```python
from build123d import *

# Parameters (mm, degrees)
F0_R     = 2.35
F0_R_2   = 0.6
F0_W     = 11.2562068871
F0_H     = 4.6791491237
F1_DEPTH = 25


with BuildPart() as f1:
    # F0 (on Top) → F1 (new body)
    with BuildSketch(Plane.XY):
        with BuildLine():
            Line((14.3979561755, 29.7439676553), (-32.8092921048, 29.7439676553))
            ThreePointArc((-32.8092921048, 29.7439676553), (-38.1665301992, 27.2495197857), (-39.7056679646, 21.5439676553))
            Line((-39.7056679646, 21.5439676553), (21.2943320354, 21.5439676553))
            ThreePointArc((21.2943320354, 21.5439676553), (19.7551942699, 27.2495197857), (14.3979561755, 29.7439676553))
        make_face()
        with Locations((-26.7056679646, 25.0439676553)):
            Circle(F0_R, mode=Mode.SUBTRACT)
        with Locations((-22.2056679646, 25.0439676553)):
            Circle(F0_R_2, mode=Mode.SUBTRACT)
        with BuildLine():
            ThreePointArc((-14.2060092107, 24.2939676534), (-14.0292525699, 24.2207333822), (-13.9560402329, 24.0439676553))
            ThreePointArc((-13.9560402329, 24.0439676553), (-14.3828278959, 23.8672019284), (-14.2060092107, 24.2939676534))
        make_face(mode=Mode.SUBTRACT)
        with BuildLine():
            ThreePointArc((-13.4558540993, 25.5439676553), (-13.6755569185, 25.0136046664), (-14.2059471661, 24.7939676611))
            ThreePointArc((-14.2059471661, 24.7939676611), (-14.9558540936, 25.5440607221), (-14.2057610325, 26.2939676495))
            ThreePointArc((-14.2057610325, 26.2939676495), (-13.6754911104, 26.0742648361), (-13.4558540993, 25.5439676553))
        make_face(mode=Mode.SUBTRACT)
        with BuildLine():
            ThreePointArc((-13.9556679658, 27.0439676553), (-14.0289022388, 26.8671799923), (-14.205698988, 26.7939676572))
            ThreePointArc((-14.205698988, 26.7939676572), (-14.3824336927, 27.2207553183), (-13.9556679658, 27.0439676553))
        make_face(mode=Mode.SUBTRACT)
        with BuildLine():
            ThreePointArc((-13.2056679646, 24.0439676553), (-12.9556679646, 24.2939676553), (-12.7056679646, 24.0439676553))
            ThreePointArc((-12.7056679646, 24.0439676553), (-12.9556679646, 23.7939676553), (-13.2056679646, 24.0439676553))
        make_face(mode=Mode.SUBTRACT)
        with BuildLine():
            ThreePointArc((-11.9557127462, 24.0439676553), (-11.7057127462, 24.2939676553), (-11.4557127462, 24.0439676553))
            ThreePointArc((-11.4557127462, 24.0439676553), (-11.7057127462, 23.7939676553), (-11.9557127462, 24.0439676553))
        make_face(mode=Mode.SUBTRACT)
        with BuildLine():
            ThreePointArc((-10.7056679646, 24.0439676553), (-10.4556679646, 24.2939676553), (-10.2056679646, 24.0439676553))
            ThreePointArc((-10.2056679646, 24.0439676553), (-10.4556679646, 23.7939676553), (-10.7056679646, 24.0439676553))
        make_face(mode=Mode.SUBTRACT)
        with BuildLine():
            ThreePointArc((-9.4556679644, 24.0439676553), (-9.2056679644, 24.2939676553), (-8.9556679644, 24.0439676553))
            ThreePointArc((-8.9556679644, 24.0439676553), (-9.2056679644, 23.7939676553), (-9.4556679644, 24.0439676553))
        make_face(mode=Mode.SUBTRACT)
        with BuildLine():
            ThreePointArc((-13.2056679651, 27.0439676553), (-12.9556679651, 27.2939676553), (-12.7056679651, 27.0439676553))
            ThreePointArc((-12.7056679651, 27.0439676553), (-12.9556679651, 26.7939676553), (-13.2056679651, 27.0439676553))
        make_face(mode=Mode.SUBTRACT)
        with BuildLine():
            ThreePointArc((-11.9556679649, 27.0439676553), (-11.7056679649, 27.2939676553), (-11.4556679649, 27.0439676553))
            ThreePointArc((-11.4556679649, 27.0439676553), (-11.7056679649, 26.7939676553), (-11.9556679649, 27.0439676553))
        make_face(mode=Mode.SUBTRACT)
        with BuildLine():
            ThreePointArc((-10.7056679648, 27.0439676553), (-10.4556679648, 27.2939676553), (-10.2056679648, 27.0439676553))
            ThreePointArc((-10.2056679648, 27.0439676553), (-10.4556679648, 26.7939676553), (-10.7056679648, 27.0439676553))
        make_face(mode=Mode.SUBTRACT)
        with BuildLine():
            ThreePointArc((-9.4556679646, 27.0439676553), (-9.2056679646, 27.2939676553), (-8.9556679646, 27.0439676553))
            ThreePointArc((-8.9556679646, 27.0439676553), (-9.2056679646, 26.7939676553), (-9.4556679646, 27.0439676553))
        make_face(mode=Mode.SUBTRACT)
        with BuildLine():
            ThreePointArc((-8.2056679646, 24.0439676553), (-7.9556679646, 24.2939676553), (-7.7056679646, 24.0439676553))
            ThreePointArc((-7.7056679646, 24.0439676553), (-7.9556679646, 23.7939676553), (-8.2056679646, 24.0439676553))
        make_face(mode=Mode.SUBTRACT)
        with BuildLine():
            ThreePointArc((-6.9557127451, 24.0439676553), (-6.7057127451, 24.2939676553), (-6.4557127451, 24.0439676553))
            ThreePointArc((-6.4557127451, 24.0439676553), (-6.7057127451, 23.7939676553), (-6.9557127451, 24.0439676553))
        make_face(mode=Mode.SUBTRACT)
        with BuildLine():
            ThreePointArc((-5.7056679646, 24.0439676553), (-5.4556679646, 24.2939676553), (-5.2056679646, 24.0439676553))
            ThreePointArc((-5.2056679646, 24.0439676553), (-5.4556679646, 23.7939676553), (-5.7056679646, 24.0439676553))
        make_face(mode=Mode.SUBTRACT)
        with BuildLine():
            ThreePointArc((-8.2056679645, 27.0439676553), (-7.9556679645, 27.2939676553), (-7.7056679645, 27.0439676553))
            ThreePointArc((-7.7056679645, 27.0439676553), (-7.9556679645, 26.7939676553), (-8.2056679645, 27.0439676553))
        make_face(mode=Mode.SUBTRACT)
        with BuildLine():
            ThreePointArc((-6.9556679644, 27.0439676553), (-6.7056679644, 27.2939676553), (-6.4556679644, 27.0439676553))
            ThreePointArc((-6.4556679644, 27.0439676553), (-6.7056679644, 26.7939676553), (-6.9556679644, 27.0439676553))
        make_face(mode=Mode.SUBTRACT)
        with BuildLine():
            ThreePointArc((-5.7056679642, 27.0439676553), (-5.4556679642, 27.2939676553), (-5.2056679642, 27.0439676553))
            ThreePointArc((-5.2056679642, 27.0439676553), (-5.4556679642, 26.7939676553), (-5.7056679642, 27.0439676553))
        make_face(mode=Mode.SUBTRACT)
        with BuildLine():
            ThreePointArc((-4.4552956958, 24.0439676553), (-4.3820723911, 24.2207443506), (-4.2052956958, 24.2939676553))
            ThreePointArc((-4.2052956958, 24.2939676553), (-4.0285190005, 24.2207443506), (-3.9552956958, 24.0439676553))
            ThreePointArc((-3.9552956958, 24.0439676553), (-4.2052956958, 23.7939676553), (-4.4552956958, 24.0439676553))
        make_face(mode=Mode.SUBTRACT)
        with BuildLine():
            ThreePointArc((-4.2052956958, 26.2927266955), (-3.6749656099, 26.0730567814), (-3.4552956958, 25.5427266955))
            ThreePointArc((-3.4552956958, 25.5427266955), (-3.6749656099, 25.0123966096), (-4.2052956958, 24.7927266955))
            ThreePointArc((-4.2052956958, 24.7927266955), (-4.9552956958, 25.5427266955), (-4.2052956958, 26.2927266955))
        make_face(mode=Mode.SUBTRACT)
        with BuildLine():
            ThreePointArc((-4.4552956958, 27.0439676553), (-4.2052956958, 27.2939676553), (-3.9552956958, 27.0439676553))
            ThreePointArc((-3.9552956958, 27.0439676553), (-4.0285190005, 26.86719096), (-4.2052956958, 26.7939676553))
            ThreePointArc((-4.2052956958, 26.7939676553), (-4.3820723911, 26.86719096), (-4.4552956958, 27.0439676553))
        make_face(mode=Mode.SUBTRACT)
        with BuildLine():
            ThreePointArc((3.1943320354, 25.0439676553), (3.7943320354, 25.6439676553), (4.3943320354, 25.0439676553))
            ThreePointArc((4.3943320354, 25.0439676553), (3.7943320354, 24.4439676553), (3.1943320354, 25.0439676553))
        make_face(mode=Mode.SUBTRACT)
        with Locations((8.2943320354, 25.0439676553)):
            Circle(F0_R, mode=Mode.SUBTRACT)
        with BuildLine():
            Line((21.2943320354, 21.5439676553), (-39.7056679646, 21.5439676553))
            ThreePointArc((-39.7056679646, 21.5439676553), (-32.2227110241, -20.6618643282), (-38.9579393192, -62.9934553426))
            ThreePointArc((-38.9579393192, -62.9934553426), (-24.3057130509, -57.6752555094), (-8.8414815134, -55.7185932914))
            ThreePointArc((-8.8414815134, -55.7185932914), (6.6735895327, -57.2197776633), (21.4758319523, -62.1049187496))
            ThreePointArc((21.4758319523, -62.1049187496), (21.0704059046, -60.8750508624), (20.6770190087, -59.6412793882))
            ThreePointArc((20.6770190087, -59.6412793882), (20.3861242332, -58.701088988), (20.102220838, -57.7587638735))
            ThreePointArc((20.102220838, -57.7587638735), (14.6254783963, -18.0161093174), (21.2943320354, 21.5439676553))
        make_face()
        with BuildLine():
            ThreePointArc((20.1618171154, -60.5971505286), (5.9837949331, -56.0337141088), (-8.8453337957, -54.6415194007))
            ThreePointArc((-8.8453337957, -54.6415194007), (-23.6223514922, -56.4857159211), (-37.6520263883, -61.4786644604))
            ThreePointArc((-37.6520263883, -61.4786644604), (-30.6700495718, -20.4154751217), (-38.3026989884, 20.5317614372))
            Line((-38.3026989884, 20.5317614372), (19.5693860733, 20.5317614372))
            ThreePointArc((19.5693860733, 20.5317614372), (12.9591755519, -20.083127629), (20.1618171154, -60.5971505286))
        make_face(mode=Mode.SUBTRACT)
        with BuildLine():
            ThreePointArc((-8.8414815134, -55.7185932914), (-24.3057130509, -57.6752555094), (-38.9579393192, -62.9934553426))
            ThreePointArc((-38.9579393192, -62.9934553426), (-36.9077506183, -67.9433195168), (-31.9579393215, -69.9936358778))
            ThreePointArc((-31.9579393215, -69.9936358778), (-8.2896342498, -67.5792618139), (15.448370366, -69.168287914))
            ThreePointArc((15.448370366, -69.168287914), (19.8018461507, -66.7798624881), (21.4758319523, -62.1049187496))
            ThreePointArc((21.4758319523, -62.1049187496), (6.6735895327, -57.2197776633), (-8.8414815134, -55.7185932914))
        make_face()
        with Locations((-8.3661192098, -62.5506510849)):
            Rectangle(F0_W, F0_H, mode=Mode.SUBTRACT)
        with BuildLine():
            Line((20.6983805739, -59.645034679), (20.102220838, -57.7587638735))
            ThreePointArc((20.102220838, -57.7587638735), (20.3861242332, -58.701088988), (20.6770190087, -59.6412793882))
            Line((20.6770190087, -59.6412793882), (20.6983805739, -59.645034679))
        make_face()
        with BuildLine():
            Line((20.6983805739, -59.645034679), (20.6770190087, -59.6412793882))
            ThreePointArc((20.6770190087, -59.6412793882), (21.0704059046, -60.8750508624), (21.4758319523, -62.1049187496))
            Line((21.4758319523, -62.1049187496), (20.6983805739, -59.645034679))
        make_face()
    extrude(amount=F1_DEPTH)


solid = f1.part
```
Design review of the part built by this model. Coordinates are the model's own, in mm. A direction names the side the tool comes from. Coordinates: 2 decimals unless noted, no trailing zeros. Order: outer loops, then holes, each group sorted by start corner. A loop starts at its lowest first (then second) coordinate and runs counter-clockwise, first axis right, second up. Notation, with made-up numbers: (15.25, 32) -> (40.25, 32) arc R31 ccw to (40.25, 69) -> close; hole circle Ø4 at (57, -10.75). An arc over 180 degrees is marked (long way). One line per item, written item: value. Start each with the question number.
Q1. For probe 1 along Y at (x, z) = (-6, 20.25); probe 2 along Y at (x, z) = (7.5, 18); probe 3 along X at (y, z) = (23, 14.25), list the stretches that pass through material, from the lowest coordinate up.
Q2. Take a section at D-D, the plane y = -4.5. State the section outline as (x, z) points, then the cut area to 3 significant figures.
Q3. Take a section at B-B, the plane x = 8.5. State the section outline as (y, z) points, then the cut area to 3 significant figures.
Q4. Tool access review of faces 4 (the flat face through (-2.738, -63, 12)), 5 (the flat face through (-32, -16, 0)): name each direction out of +Z, -Z, +X, -X, +Y, -Y from which nothing blocks a thin tool from reaching the whole face with its end or side.
Q5. Take a section at A-A, the plane y = 14.5. State the section outline as (x, z) points, then the cut area to 3 significant figures.
Q6. Insertion check: pin 1 Ø7.5 at (x, z) = (-5, 7) entering from -Y; pin 2 Ø2.5 at (y, z) = (-61.5, 15) entering from -X; pin 3 Ø1.5 at (x, y) = (-30.5, 19.5) entering from +Z; pin 4 Ø2 at (x, z) = (14.5, 15.5) entering from -Y. Each pin has a flat end and moves straight along its axis. Give the tip position at first contact, or say it passes through.
Q7. Mouldability with a two-part tool opening along X and no side actions: class faces 1 (the flat face through (-9, 29.744, 12)), 2 (the flat face through (-10, 20.532, 12)), 3 (the cylindrical face through (-38.111, 27.315, 12.325)) as pulls with the +X half, pulls with the -X half, needs draft (parallel to the pull), parting line crosses it, or undercut.
Q8. Take a section at C-C, the plane z = 18.75. Give the number of separate pieces and of enclosed holes in the cut face, then the cut area to 3 significant figures.
Values follow:
1. probe 1: y = -67.56 to -64.89, -60.21 to -54.66, 20.53 to 29.74
1. probe 2: y = -68.19 to -56.36, 20.53 to 22.83, 27.26 to 29.74
1. probe 3: x = -39.8 to -27.87, -25.55 to 7.13, 9.45 to 21.39
2. outline: (-33.38, 0) -> (-31.87, 0) -> (-31.87, 25) -> (-33.38, 25) -> close; (13.84, 0) -> (15.52, 0) -> (15.52, 25) -> (13.84, 25) -> close
2. area: 79.9 mm2
3. outline: (-68.29, 0) -> (-56.6, 0) -> (-56.6, 25) -> (-68.29, 25) -> close; (20.53, 0) -> (22.7, 0) -> (22.7, 25) -> (20.53, 25) -> close; (27.38, 0) -> (29.74, 0) -> (29.74, 25) -> (27.38, 25) -> close
3. area: 405 mm2
4. face 4: +Z, -Z
4. face 5: -Z, +X, -X, +Y, -Y
5. outline: (-37.42, 0) -> (-36.21, 0) -> (-36.21, 25) -> (-37.42, 25) -> close; (17.68, 0) -> (19.18, 0) -> (19.18, 25) -> (17.68, 25) -> close
5. area: 68.0 mm2
6. pin 1: stops at y = -67.63
6. pin 2: stops at x = -38.88
6. pin 3: passes through
6. pin 4: stops at y = -69.17
7. face 1: needs draft
7. face 2: undercut
7. face 3: pulls with the -X half
8. separate pieces: 1
8. enclosed holes: 26
8. area: 1,360 mm2
